The listing builds one solid part. Answer for the finished solid, in the listing's coordinates (mm). Give positions to 0.01 mm unless a question says otherwise; leave off trailing zeros. Write each loop counter-clockwise with the first axis right and the second up, starting at its lowest first coordinate (ties: lowest second). Pieces come first, ordered by that corner, then holes. Notation, with made-up numbers: M 71,12.5 L 97,12.5 A15 cw 97,17.5 Z; hole C -35.75,-1 d10. An arc over 180 degrees is marked long. Return JSON: item names as keys, results as strings.
from build123d import *

# Parameters (mm, degrees)
SKETCH1_W           = 25.15
SKETCH1_H           = 22.4
SKETCH1_R           = 1.25
SKETCH1_R_2         = 0.5
BOSS_EXTRUDE1_DEPTH = 1.6


with BuildPart() as part:
    # Sketch1 → Boss-Extrude1 (new body)
    with BuildSketch(Plane.XY):
        Rectangle(SKETCH1_W, SKETCH1_H)
        with Locations((-10.1, 8.6)):
            Circle(SKETCH1_R, mode=Mode.SUBTRACT)
        with Locations((10.1, 8.6)):
            Circle(SKETCH1_R, mode=Mode.SUBTRACT)
        with Locations((-10.1, -8.6)):
            Circle(SKETCH1_R, mode=Mode.SUBTRACT)
        with Locations((10.1, -8.6)):
            Circle(SKETCH1_R, mode=Mode.SUBTRACT)
        with Locations((-1.75, 8.2)):
            Circle(SKETCH1_R_2, mode=Mode.SUBTRACT)
        with Locations((1.75, 8.2)):
            Circle(SKETCH1_R_2, mode=Mode.SUBTRACT)
        with Locations((-6.075, -8.7)):
            Circle(SKETCH1_R_2, mode=Mode.SUBTRACT)
        with Locations((-3.535, -8.7)):
            Circle(SKETCH1_R_2, mode=Mode.SUBTRACT)
        with Locations((-0.995, -8.7)):
            Circle(SKETCH1_R_2, mode=Mode.SUBTRACT)
        with Locations((1.545, -8.7)):
            Circle(SKETCH1_R_2, mode=Mode.SUBTRACT)
        with Locations((4.085, -8.7)):
            Circle(SKETCH1_R_2, mode=Mode.SUBTRACT)
        with Locations((6.625, -8.7)):
            Circle(SKETCH1_R_2, mode=Mode.SUBTRACT)
    extrude(amount=BOSS_EXTRUDE1_DEPTH)


solid = part.part
Item 1: A cutting plane is placed at A-A, the plane x = -10.1. Write down the section's boundary in (y, z), plus the area to 3 significant figures.
Geometry results:
{"outline": "M -11.2,0 L -9.85,0 L -9.85,1.6 L -11.2,1.6 Z; M -7.35,0 L 7.35,0 L 7.35,1.6 L -7.35,1.6 Z; M 9.85,0 L 11.2,0 L 11.2,1.6 L 9.85,1.6 Z", "area": "27.8 mm2"}
Item 2: Determine the mould class of faces 1 (the cylindrical face through (1.18, -8.36, 0.79)), 2 (the flat face through (12.575, 0, 1)), 3 (the flat face through (0, 0, 0)) for opening direction X: +X half, -X half, draft (parallel to the pull), parting line (faces both ways), or undercut.
Geometry results:
{"face 1": "undercut", "face 2": "+X half", "face 3": "draft"}
Item 3: A cutting plane is placed at B-B, the plane z = 0.8. Count the separate pieces of the cut face and the enclosed holes in it, plus the area to 3 significant figures.
Geometry results:
{"separate pieces": "1", "enclosed holes": "12", "area": "537 mm2"}
Item 4: A cutting plane is placed at C-C, the plane y = 9.5. Write down the section's boundary in (x, z) (3 decimals).
Geometry results:
{"outline": "M -12.575,0 L -10.967,0 L -10.967,1.6 L -12.575,1.6 Z; M -9.233,0 L 9.233,0 L 9.233,1.6 L -9.233,1.6 Z; M 10.967,0 L 12.575,0 L 12.575,1.6 L 10.967,1.6 Z"}
Item 5: Find the intervals of material crossed by line 1 (Y direction, x = 10.1, z = 0.95); line 2 (X direction, y = 9, z = 0.4) (3 decimals); line 3 (Y direction, x = 4, z = 0.95), in increasing order.
Geometry results:
{"line 1": "y = -11.2 to -9.85, -7.35 to 7.35, 9.85 to 11.2", "line 2": "x = -12.575 to -11.284, -8.916 to 8.916, 11.284 to 12.575", "line 3": "y = -11.2 to -9.19, -8.21 to 11.2"}
